Autodesk Inventor part; units mm, degrees
ref_plane "YZ Plane" through (0, 0, 0) normal (1, 0, 0) x (0, 1, 0)
ref_plane "XZ Plane" through (0, 0, 0) normal (0, 1, 0) x (-1, 0, 0)
ref_plane "XY Plane" through (0, 0, 0) normal (0, 0, 1) x (1, 0, 0)
sketch "Sketch1" plane through (0, 0, 0) normal (0, 0, 1) x (1, 0, 0)
  line L0 (-2.5, 15.5) -> (2.5, 15.5)
  line L1 (2.5, 15.5) -> (2.5, -4.5)
  line L2 (2.5, -4.5) -> (-2.5, -4.5)
  line L3 (-2.5, -4.5) -> (-2.5, 15.5)
  point P0 (0, 0)
  dimension "d0" = 5
  dimension "d1" = 20
extrude "Extrusion1" add sketch "Sketch1" along normal blind 40
sketch "Sketch3" plane through (-2.5, -4.5, 0) normal (-1, 0, 0) x (0, 0, 1)
  line L0 (0, 0) -> (0, 20)
  line L1 (0, 10) -> (2.5, 10)
  line L2 (2.5, 10) -> (7.5, 10)
  circle A0 centre (7.5, 10) radius 4.75
  point P0 (0, 4.5)
  dimension "d7" = 2.5
  dimension "d38" = 5
  dimension "d39" = 9.5
extrude "Extrusion2" cut sketch "Sketch3" against normal blind 8
sketch "Sketch4" plane through (-2.5, -4.5, 0) normal (-1, 0, 0) x (0, 0, 1)
  line L0 (40, 0) -> (40, 20)
  line L1 (40, 0) -> (30, 0)
  line L2 (30, 0) -> (30, 0.8)
  line L3 (30, 0.8) -> (40, 0.8)
  line L4 (40, 0.8) -> (40, 0)
  line L5 (40, 0.8) -> (40, 2)
  line L6 (40, 2) -> (30, 2)
  line L7 (30, 2) -> (30, 2.8)
  line L8 (30, 2.8) -> (40, 2.8)
  line L9 (40, 2.8) -> (40, 2)
  line L10 (40, 2.8) -> (40, 4)
  line L11 (40, 4) -> (30, 4)
  line L12 (30, 4) -> (30, 4.8)
  line L13 (30, 4.8) -> (40, 4.8)
  line L14 (40, 4.8) -> (40, 4)
  line L15 (40, 4.8) -> (40, 6)
  line L16 (40, 6) -> (30, 6)
  line L17 (30, 6) -> (30, 6.8)
  line L18 (30, 6.8) -> (40, 6.8)
  line L19 (40, 6.8) -> (40, 6)
  line L20 (40, 6.8) -> (40, 8)
  line L21 (40, 8) -> (30, 8)
  line L22 (30, 8) -> (30, 8.8)
  line L23 (30, 8.8) -> (40, 8.8)
  line L24 (40, 8.8) -> (40, 8)
  line L25 (40, 8.8) -> (40, 10)
  line L26 (40, 10) -> (30, 10)
  line L27 (30, 10) -> (30, 10.8)
  line L28 (30, 10.8) -> (40, 10.8)
  line L29 (40, 10.8) -> (40, 10)
  line L30 (40, 10.8) -> (40, 12)
  line L31 (40, 12) -> (30, 12)
  line L32 (30, 12) -> (30, 12.8)
  line L33 (30, 12.8) -> (40, 12.8)
  line L34 (40, 12.8) -> (40, 12)
  line L35 (40, 12.8) -> (40, 14)
  line L36 (40, 14) -> (30, 14)
  line L37 (30, 14) -> (30, 14.8)
  line L38 (30, 14.8) -> (40, 14.8)
  line L39 (40, 14.8) -> (40, 14)
  line L40 (40, 14.8) -> (40, 16)
  line L41 (40, 16) -> (30, 16)
  line L42 (30, 16) -> (30, 16.8)
  line L43 (30, 16.8) -> (40, 16.8)
  line L44 (40, 16.8) -> (40, 16)
  line L45 (40, 16.8) -> (40, 18)
  line L46 (40, 18) -> (30, 18)
  line L47 (30, 18) -> (30, 18.8)
  line L48 (30, 18.8) -> (40, 18.8)
  line L49 (40, 18.8) -> (40, 18)
  point P0 (0, 4.5)
  dimension "d12" = 10
  dimension "d13" = 0.8
  dimension "d14" = 1.2
  dimension "d15" = 0.8
  dimension "d16" = 1.2
  dimension "d17" = 0.8
  dimension "d18" = 1.2
  dimension "d19" = 0.8
  dimension "d20" = 1.2
  dimension "d21" = 0.8
  dimension "d22" = 1.2
  dimension "d29" = 0.8
  dimension "d30" = 1.2
  dimension "d31" = 0.8
  dimension "d32" = 1.2
  dimension "d33" = 0.8
  dimension "d34" = 1.2
  dimension "d35" = 0.8
  dimension "d36" = 1.2
  dimension "d37" = 0.8
extrude "Extrusion3" add sketch "Sketch4" along normal blind 2
sketch "Sketch5" plane through (-2.5, -4.5, 0) normal (-1, 0, 0) x (0, 0, 1)
  circle A0 centre (7.5, 10) radius 4.75
  line L0 (12.4308, 11.5) -> (18, 11.5)
  line L1 (22.4308, 8.5) -> (22.4308, 11.5)
  line L2 (22.4308, 11.5) -> (18, 11.5)
  line L3 (22.4308, 8.5) -> (11.2154, 8.5)
  line L4 (11.2154, 8.5) -> (11.2154, 11.5)
  line L5 (11.2154, 11.5) -> (12.4308, 11.5)
  point P0 (0, 4.5)
extrude "Extrusion4" cut sketch "Sketch5" against normal blind 40 contours A0 L3 L4 L5 | A0 L5 L0 L2 L1 L3 picked at (11.5603, 10)
sketch "Sketch6" plane through (-2.5, 15.5, 0) normal (0, 1, 0) x (1, 0, 0)
  line L0 (0, 0) -> (0, -40)
  line L1 (0, -15.1532) -> (2.5, -15.1532)
  point P0 (2.5, 0)
hole "Hole1" at (0, 15.5, 15.1532) direction (0, -1, 0) diameter 3.1 depth 49.5
sketch "Sketch7" plane through (0, 0, 0) normal (0, 0, -1) x (-1, 0, 0)
  line L0 (-2.5, -4.5) -> (-2.5, 15.5)
  line L1 (-2.5, 15.5) -> (2.5392, 15.5)
  line L2 (2.5392, 15.5) -> (2.5392, -4.5)
  line L3 (2.5392, -4.5) -> (-2.5, -4.5)
  line L4 (-2.5, -4.5) -> (-2.5, 15.5)
  point P0 (0, 0)
extrude "Extrusion5" cut sketch "Sketch7" against normal blind 0.4
properties part number "teethset"
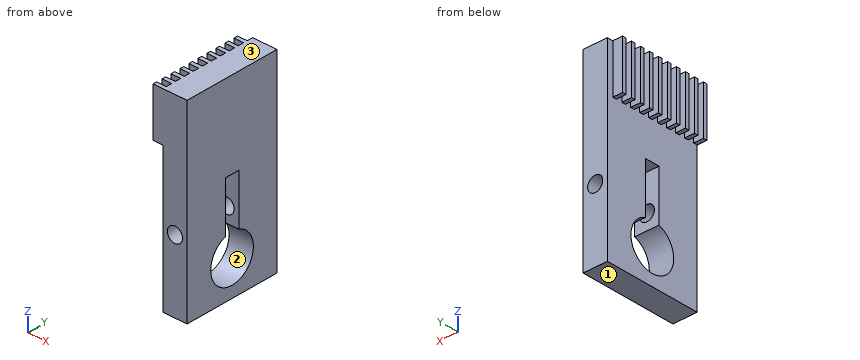
Could you check a few things on this model? Use its own coordinates, in mm. Face numbers are marked on the shaded views. Round coordinates to 2 decimals unless told otherwise and drop trailing zeros. Order: outer loops, then holes, each group sorted by start corner. A loop starts at its lowest first (then second) coordinate and runs counter-clockwise, first axis right, second up.
Q1. I'm going to push flat-ended pins straight in: P1, Ø0.9, axis at x = -3.5, y = 12, coming from the -Z side; P2, Ø1, axis at x = -3.5, z = 33, coming from the +Y side; P3, Ø12, axis at y = 6, z = 11, coming from the -X side. Where does each tip first touch, or does it pass through?
Geometry says:
P1: stops at z = 30
P2: stops at y = 14.3
P3: stops at x = -2.5
Q2. Please list where these lines run through material, in increasing order: probe 1 along Z at (x, y) = (0, -2.25); probe 2 along Y at (x, z) = (-1.45, 7.5); probe 3 along Y at (x, z) = (2.25, 20).
Geometry says:
probe 1: z = 0.4 to 13.6, 16.7 to 40
probe 2: y = -4.5 to 0.75, 10.25 to 15.5
probe 3: y = -4.5 to 4, 7 to 15.5
Q3. Imagine slicing it at B-B, the plane y = 9. List the corners of the cut face in (x, z) for me.
Geometry says:
outline: (-2.5, 0.4) - (2.5, 0.4) - (2.5, 4.29) - (-2.5, 4.29) - close; (-2.5, 10.71) - (2.5, 10.71) - (2.5, 40) - (-2.5, 40) - close; hole circle Ø3.1 at (0, 15.15)
Q4. Imagine slicing it at D-D, the plane y = 4.75. List the corners of the cut face in (x, z) for me, then the cut area to 3 significant figures.
Geometry says:
outline: (-2.5, 0.4) - (2.5, 0.4) - (2.5, 2.81) - (-2.5, 2.81) - close; (-2.5, 22.43) - (2.5, 22.43) - (2.5, 40) - (-2.5, 40) - close
area: 99.9 mm2
Q5. Thinking about a two-plate mould opening in Z: for the marked faces 1, 2 and 3, which applies, released by +Z, released by -Z, zero draft, split by the parting line, or undercut?
Geometry says:
face 1: released by -Z
face 2: undercut
face 3: released by +Z
Q6. Imagine slicing it at A-A, the plane z = 17.5. List the corners of the cut face in (x, y) for me.
Geometry says:
outline: (-2.5, -4.5) - (2.5, -4.5) - (2.5, 4) - (-2.5, 4) - close; (-2.5, 7) - (2.5, 7) - (2.5, 15.5) - (-2.5, 15.5) - close
Q7. Imagine slicing it at C-C, the plane x = 0. List the corners of the cut face in (y, z) for me.
Geometry says:
outline: (-4.5, 0.4) - (15.5, 0.4) - (15.5, 13.6) - (7, 13.6) - (7, 12.01) arc R4.75 cw (long way) to (4, 12.01) - (4, 13.6) - (-4.5, 13.6) - close; (-4.5, 16.7) - (4, 16.7) - (4, 22.43) - (7, 22.43) - (7, 16.7) - (15.5, 16.7) - (15.5, 40) - (-4.5, 40) - close
